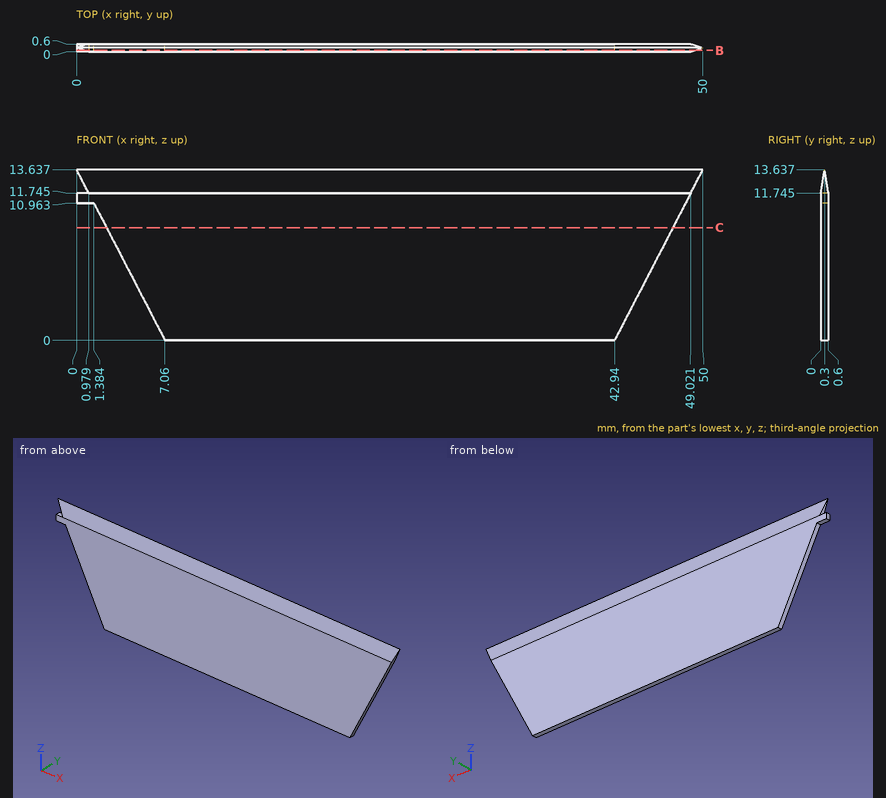
The drawing under review shows one solid part. Ordinate dimensions are in mm from its lowest x, y, z. Coordinates: 2 decimals unless noted, no trailing zeros. Order: outer loops, then holes, each group sorted by start corner. A loop starts at its lowest first (then second) coordinate and runs counter-clockwise, first axis right, second up. Notation, with made-up numbers: M 37.5,-27 L 67.5,-27 A17 ccw 67.5,5 Z; hole C 78.25,65 d9. An arc over 180 degrees is marked long. Use a Markdown table: item, result.
(1) Add section B-B (y = 0.1). Give the boundary of the cut face in (x, z) (1 decimal).
Worked answers:
| item | result |
|---|---|
| outline | M 0,11 L 1.4,11 L 7.1,0 L 42.9,0 L 49.3,12.4 L 0.7,12.4 L 1,11.7 L 0,11.7 Z |
(2) Add section C-C (z = 9). Give the boundary of the cut face in (x, y).
Worked answers:
| item | result |
|---|---|
| outline | M 2.4,0 L 47.6,0 L 47.6,0.6 L 2.4,0.6 Z |
(3) Wall thickness on probe 1 along X at (y, z) = (0.1, 3.5); probe 2 along X at (y, z) = (0.3, 8); probe 3 along Y at (x, z) = (13, 13): over which ranges is each line inside the solid? List them lowest first.
Worked answers:
| item | result |
|---|---|
| probe 1 | x = 5.25 to 44.75 |
| probe 2 | x = 2.92 to 47.08 |
| probe 3 | y = 0.2 to 0.4 |
